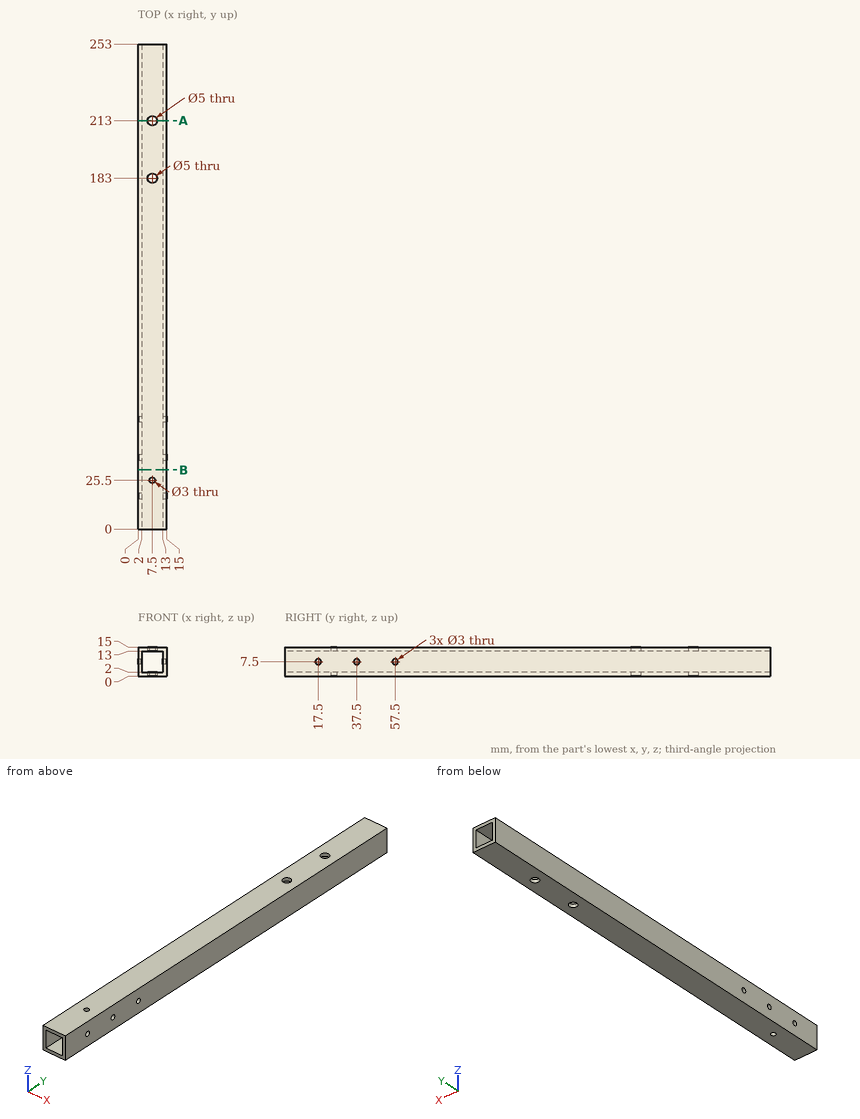
Print and shaded views of the part. All mm, measured from the part's lowest x, y and z. Give positions to 0.01 mm unless a question says otherwise; leave off trailing zeros. Order: outer loops, then holes, each group sorted by start corner. A loop starts at its lowest first (then second) coordinate and runs counter-clockwise, first axis right, second up. Notation, with made-up numbers: M 32,69 L 72,69 A14 ccw 72,73 Z; hole C 40,81.25 d10. An arc over 180 degrees is marked long. Use one line per item in the form item = value.
Q1. Slice it at B-B, the plane y = 31. Write the cut outline in (x, z).
Conclusion:
outline = M 0,0 L 15,0 L 15,15 L 0,15 Z; hole M 2,2 L 13,2 L 13,13 L 2,13 Z
Q2. Slice it at A-A, the plane y = 213. Write the cut outline in (x, z).
Conclusion:
outline = M 0,0 L 5,0 L 5,2 L 2,2 L 2,13 L 5,13 L 5,15 L 0,15 Z; M 10,0 L 15,0 L 15,15 L 10,15 L 10,13 L 13,13 L 13,2 L 10,2 Z
Q3. Wall check: probe 1 along Y at (x, z) = (14.1, 7.5); probe 2 along Y at (x, z) = (7.5, 13.75); probe 3 along Z at (x, y) = (12.5, 141). Give the ranges that are in metal, low to high.
Conclusion:
probe_1 = 0 to 16, 19 to 36, 39 to 56, 59 to 253
probe_2 = 0 to 24, 27 to 180.5, 185.5 to 210.5, 215.5 to 253
probe_3 = 0 to 2, 13 to 15
Q4. Pin check, flat tips, straight feed: P1, Ø2.5, axis at y = 37.5, z = 7.5, coming from the +X side; P2, Ø1.5, axis at y = 191, z = 3.5, coming from the -X side. Stop position of each tip, or through.
Conclusion:
P1 = through
P2 = 0
